Print and shaded views of the part. All mm, measured from the part's lowest x, y and z. Coordinates: 2 decimals unless noted, no trailing zeros. Order: outer loops, then holes, each group sorted by start corner. A loop starts at its lowest first (then second) coordinate and runs counter-clockwise, first axis right, second up. Notation, with made-up numbers: M 77,37.5 L 87,37.5 A24 cw 87,75.5 Z; hole C -33.75,33.5 d11. An arc over 180 degrees is marked long. Return JSON: item names as keys, results as strings.
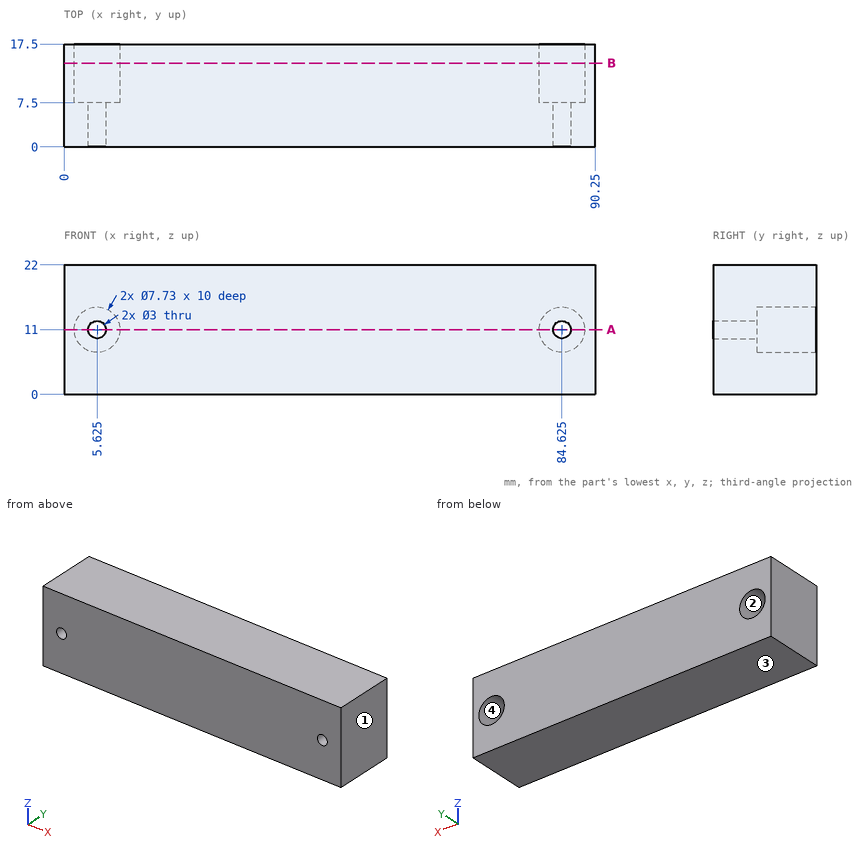
Item 1: Drop flat-ended pins along their axis: pin 1 Ø2 at (y, z) = (2, 18) entering from -X; pin 2 Ø3.5 at (x, z) = (5.625, 11) entering from +Y. Give the stop position or say it passes through.
Check result:
{"pin 1": "stops at x = 0", "pin 2": "stops at y = 7.5"}
Item 2: Saw through at A-A (z = 11). Write the cut outline in (x, y) (3 decimals).
Check result:
{"outline": "M 0,0 L 4.125,0 L 4.125,7.5 L 1.76,7.5 L 1.76,17.5 L 0,17.5 Z; M 7.125,0 L 83.125,0 L 83.125,7.5 L 80.76,7.5 L 80.76,17.5 L 9.49,17.5 L 9.49,7.5 L 7.125,7.5 Z; M 86.125,0 L 90.25,0 L 90.25,17.5 L 88.49,17.5 L 88.49,7.5 L 86.125,7.5 Z"}
Item 3: Wall check: line 1 (X direction, y = 14.5, z = 11); line 2 (X direction, y = 5.75, z = 11) (3 decimals); line 3 (Z direction, x = 85, y = 10.5). Give the ranges that are in metal, low to high.
Check result:
{"line 1": "x = 0 to 1.76, 9.49 to 80.76, 88.49 to 90.25", "line 2": "x = 0 to 4.125, 7.125 to 83.125, 86.125 to 90.25", "line 3": "z = 0 to 7.15, 14.85 to 22"}
Item 4: Pull direction Z, two halves, no side cores. Call the marked faces 1, 2, 3 and 4: +Z half, -Z half, draft (parallel to the pull), parting line (faces both ways), or undercut.
Check result:
{"face 1": "draft", "face 2": "undercut", "face 3": "-Z half", "face 4": "undercut"}
Item 5: Saw through at B-B (y = 14.25). Write the cut outline in (x, z) (3 decimals), and give its area (3 significant figures).
Check result:
{"outline": "M 0,0 L 90.25,0 L 90.25,22 L 0,22 Z; hole C 5.625,11 d7.73; hole C 84.625,11 d7.73", "area": "1,890 mm2"}
